Model file for the job. Use its own axes, mm. Face numbers are marked on the shaded views. A direction names the side the tool comes from. Round coordinates to 2 decimals unless told otherwise and drop trailing zeros. Write each loop counter-clockwise with the first axis right and the second up, starting at its lowest first coordinate (ties: lowest second). Pieces come first, ordered by that corner, then holes.
```python
from build123d import *

# Parameters (mm, degrees)
SZKIC1_R                    = 13.2
SZKIC1_R_2                  = 7.5
DODANIE_WYCI_GNI_CIE1_DEPTH = 44
DODANIE_WYCI_GNI_CIE2_DEPTH = 12
SFAZOWANIE1_SIZE            = 4
SZKIC8_R                    = 7.5
WYTNIJ_WYCI_GNI_CIE1_DEPTH  = 12
SFAZOWANIE2_SIZE            = 4


with BuildPart() as part:
    # Szkic1 → Dodanie-wyciągnięcie1 (new body)
    with BuildSketch(Plane(origin=(0, 0, 0), x_dir=(0, 0, -1), z_dir=(1, 0, 0))):
        Circle(SZKIC1_R)
        Circle(SZKIC1_R_2, mode=Mode.SUBTRACT)
    extrude(amount=DODANIE_WYCI_GNI_CIE1_DEPTH)

    # Szkic6 → Dodanie-wyciągnięcie2 (add)
    with BuildSketch(Plane(origin=(15, 0, 0), x_dir=(0, 0, -1), z_dir=(1, 0, 0))):
        Polygon((18.475208614, 0), (9.237604307, 16), (-9.237604307, 16), (-18.475208614, 0), (-9.237604307, -16), (9.237604307, -16), align=None)
    extrude(amount=DODANIE_WYCI_GNI_CIE2_DEPTH)

    # Sfazowanie1
    sfazowanie1_edges = [part.edges().sort_by_distance(p)[0] for p in [
        (44, 0, 7.5),
    ]]
    chamfer(sfazowanie1_edges, length=SFAZOWANIE1_SIZE)

    # Szkic8 → Wytnij-wyciągnięcie1 (cut)
    with BuildSketch(Plane.ZY.offset(-15)):
        with Locations(Location((0, 0, 0), (0, 0, 180))):
            Circle(SZKIC8_R)
    extrude(amount=-WYTNIJ_WYCI_GNI_CIE1_DEPTH, mode=Mode.SUBTRACT)

    # Sfazowanie2
    sfazowanie2_edges = [part.edges().sort_by_distance(p)[0] for p in [
        (0, 0, 7.5),
    ]]
    chamfer(sfazowanie2_edges, length=SFAZOWANIE2_SIZE)


solid = part.part
```
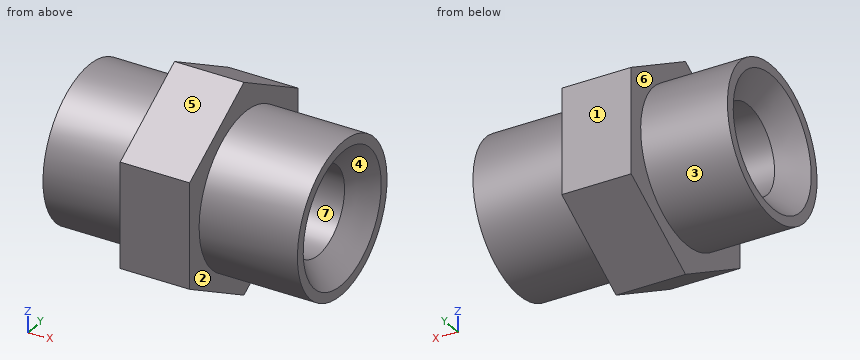
1) Flat gauge pins, fed straight in: pin 1 Ø4 at (x, y) = (15.5, -3) entering from +Z; pin 2 Ø1.5 at (x, y) = (13.5, -13) entering from +Z; pin 3 Ø12 at (y, z) = (1.5, 0.5) entering from +X. Where does each tip first touch, or does it go through?
2) Wall check: probe 1 along Y at (x, z) = (28, 0); probe 2 along Y at (x, z) = (22, 0); probe 3 along X at (y, z) = (8, -13). Give the ranges that are in metal, low to high.
3) Cut at B-B on x = 6. List the corners of the cut face in (y, z).
4) Cut at A-A on z = 0. List the corners of the cut face in (x, y).
5) Which spindle directions (+Z, -Z, +X, -X, +Y, -Y) get a long thin tool onto all of the face, cutting with end or side? Do the marked faces 1, 2 and 3. Say none if no direction does.
6) Cut at C-C on z = 15. List the corners of the cut face in (x, y).
7) Pull direction Z, two halves, no side cores. Call the marked faces 4, 5, 6 and 7: released by +Z, released by -Z, zero draft, split by the parting line, or undercut.
Result sheet:
1. pin 1: stops at z = 17.9
1. pin 2: stops at z = 4.92
1. pin 3: stops at x = 40.08
2. probe 1: y = -13.2 to -7.5, 7.5 to 13.2
2. probe 2: y = -16 to -7.5, 7.5 to 16
2. probe 3: x = 15 to 27
3. outline: circle Ø26.4 at (0, 0); hole circle Ø15 at (0, 0)
4. outline: (0, -13.2) - (15, -13.2) - (15, -16) - (27, -16) - (27, -13.2) - (44, -13.2) - (44, -11.5) - (40, -7.5) - (4, -7.5) - (0, -11.5) - close; (0, 11.5) - (4, 7.5) - (40, 7.5) - (44, 11.5) - (44, 13.2) - (27, 13.2) - (27, 16) - (15, 16) - (15, 13.2) - (0, 13.2) - close
5. face 1: +Z, -Z, +X, -X, +Y
5. face 2: +X
5. face 3: -X
6. outline: (15, -6.02) - (27, -6.02) - (27, 6.02) - (15, 6.02) - close
7. face 4: undercut
7. face 5: released by +Z
7. face 6: zero draft
7. face 7: undercut
